Geometry: final body of the model. Coordinates: model frame, mm. Give positions to 0.01 mm unless a question says otherwise; leave off trailing zeros. Order: outer loops, then holes, each group sorted by start corner. A loop starts at its lowest first (then second) coordinate and runs counter-clockwise, first axis right, second up. Notation, with made-up numbers: M 29.5,22 L 38.5,22 A11 cw 38.5,42 Z; hole C -3.5,56 d1. An arc over 180 degrees is marked long. Use CSV: the item, a comma, the result in double quotes.
Autodesk Inventor part; units mm, degrees
ref_plane "YZ Plane" through (0, 0, 0) normal (1, 0, 0) x (0, 1, 0)
ref_plane "XZ Plane" through (0, 0, 0) normal (0, 1, 0) x (-1, 0, 0)
ref_plane "XY Plane" through (0, 0, 0) normal (0, 0, 1) x (1, 0, 0)
sketch "スケッチ1" plane through (0, 0, 0) normal (0, 0, 1) x (1, 0, 0)
  line L0 (0, 16.5) -> (26, 16.5)
  line L1 (26, 16.5) -> (26, 0)
  line L2 (26, 0) -> (0, 0)
  line L3 (0, 0) -> (0, 16.5)
  circle A0 centre (13, 16.5) radius 13
  circle A1 centre (13, 16.5) radius 4.25
  circle A2 centre (13, 16.5) radius 6
  circle A3 centre (13, 22.5) radius 1
  circle A4 centre (8.7574, 20.7426) radius 1
  circle A5 centre (7, 16.5) radius 1
  circle A6 centre (8.7574, 12.2574) radius 1
  circle A7 centre (13, 10.5) radius 1
  circle A8 centre (17.2426, 12.2574) radius 1
  circle A9 centre (19, 16.5) radius 1
  circle A10 centre (17.2426, 20.7426) radius 1
  point P0 (0, 16.5)
  point P1 (26, 16.5)
  dimension "d3" = 12
  dimension "d0" = 16.5
  dimension "d1" = 26
  dimension "d2" = 8.5
  dimension "d4" = 2
  dimension "d7" = 360
extrude "押し出し1" add sketch "スケッチ1" along normal blind 1.5 contours A9 A2 A10 A3 A4 A5 L0 A0 | L0 A0 A5 A2 A6 A7 A8 A9 | A9 A2 A8 A7 A6 A5 L0 A1 | L0 A1 A5 A2 A4 A3 A10 A9 | L1 L2 L3 A0
sketch "スケッチ2" plane through (0, 0, 1.5) normal (0, 0, 1) x (1, 0, 0)
  circle A0 centre (2, 5.5906) radius 0.8
  circle A1 centre (5, 2) radius 0.8
  circle A2 centre (21, 2) radius 0.8
  circle A3 centre (13, 16.5) radius 4.25
  circle A4 centre (13, 16.5) radius 10
  line L0 (0, 0) -> (26, 0)
  line L1 (8, 7.8397) -> (8, 0)
  line L2 (18, 7.8397) -> (18, 0)
  point P0 (2, 0)
  point P1 (24, 0)
  dimension "d14" = 20
  dimension "d16" = 3
  dimension "d17" = 3
extrude "押し出し2" cut sketch "スケッチ2" against normal through all contours A0 | A1 | A2 | A4 L2 L0 L1
fillet "フィレット2" radius 3 6 edges at (0, 0, 0.75) (8, 0, 0.75) (8, 7.8397, 0.75) (18, 7.8397, 0.75) (18, 0, 0.75) (26, 0, 0.75)
properties part number "hipjoint_toleg_upper" material "アルミニウム 6061"
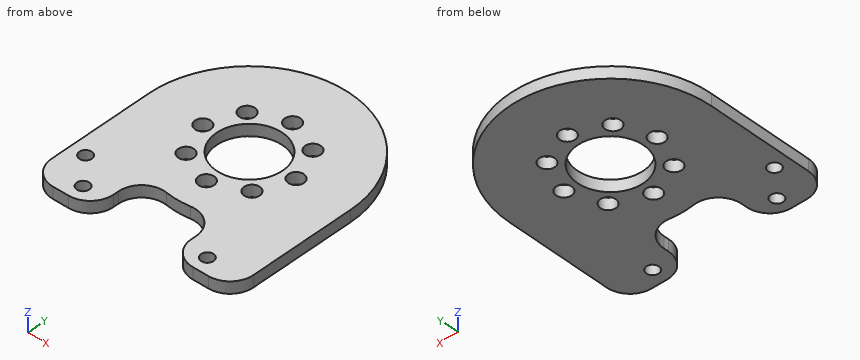
1. Section C-C, the plane y = 2. Return the cut outline in (x, z).
Answer:
outline,"M 0.17,0 L 4.2,0 L 4.2,1.5 L 0.17,1.5 Z; M 5.8,0 L 7.83,0 L 7.83,1.5 L 5.8,1.5 Z; M 18.17,0 L 20.2,0 L 20.2,1.5 L 18.17,1.5 Z; M 21.8,0 L 25.83,0 L 25.83,1.5 L 21.8,1.5 Z"
2. Pin query (flat end, axial travel): pin 1 Ø2 at (x, y) = (21, 2) entering from +Z. Return the tip coordinate at first contact, or that it passes through.
Answer:
pin 1,"z = 1.5"
3. Line query: line 1 (X direction, y = 3.25, z = 0.1); line 2 (X direction, y = 21, z = 0.6); line 3 (X direction, y = 15.75, z = 1.2). Output: solid intervals per line, ascending.
Answer:
line 1,"0 to 8, 18 to 26"
line 2,"0.8 to 7.79, 9.72 to 16.28, 18.21 to 25.2"
line 3,"0 to 6.34, 7.66 to 8.82, 17.18 to 18.34, 19.66 to 26"
4. Section B-B, the plane x = 19. Return the cut outline in (y, z).
Answer:
outline,"M 0.76,0 L 15.5,0 L 15.5,1.5 L 0.76,1.5 Z; M 17.5,0 L 28.03,0 L 28.03,1.5 L 17.5,1.5 Z"
5. Section A-A, the plane y = 10.5. Return the cut outline in (x, z).
Answer:
outline,"M 0,0 L 12,0 L 12,1.5 L 0,1.5 Z; M 14,0 L 26,0 L 26,1.5 L 14,1.5 Z"
6. Section D-D, the plane z = 0.65. Give the number of separate pieces and of enclosed holes in the cut face, plus the area to 3 significant figures.
Answer:
separate pieces,"1"
enclosed holes,"12"
area,"537 mm2"
